from build123d import *

# Parameters (mm, degrees)
CHAMFER8_SIZE       = 0.55
BOSS_EXTRUDE3_START = 3
SKETCH8_R           = 3.9
BOSS_EXTRUDE3_DEPTH = 3


with BuildPart() as part:
    # Sketch1 → Revolve1 (revolve)
    with BuildSketch(Plane(origin=(0, 0, 0), x_dir=(1, 0, 0), z_dir=(0, 1, 0)), mode=Mode.PRIVATE) as revolve1_sk:
        Polygon((-11.4, 3.1), (11.4, 3.1), (11.4, 3.9), (4.4, 3.9), (4.4, 5), (-4.4, 5), (-4.4, 3.9), (-11.4, 3.9), align=None)
    revolve(revolve1_sk.sketch.rotate(Axis((-11.4, 0, 0), (1, 0, 0)), 180), axis=Axis((-11.4, 0, 0), (1, 0, 0)))

    # Chamfer8
    chamfer8_edges = [part.edges().sort_by_distance(p)[0] for p in [
        (4.4, 0, -3.9),
        (4.4, 0, -5),
        (-4.4, 0, -5),
        (-4.4, 0, -3.9),
    ]]
    chamfer(chamfer8_edges, length=CHAMFER8_SIZE - 0.0001)  # a hair under: the kernel refuses the full size

    # Sketch8 → Boss-Extrude3 (add)
    with BuildSketch(Plane.ZY.offset(11.4).offset(BOSS_EXTRUDE3_START)):
        Circle(SKETCH8_R)
    extrude(amount=-BOSS_EXTRUDE3_DEPTH)


solid = part.part
Design review of the part built by this model. Coordinates are the model's own, in mm. A direction names the side the tool comes from. Give positions to 0.01 mm unless a question says otherwise; leave off trailing zeros. Loops run counter-clockwise (first coordinate to the right, second up) from the corner with the lowest first, then second, coordinate; pieces in that order, holes last. Notation, with made-up numbers: M 70.5,48.25 L 106.5,48.25 A26 cw 106.5,69.25 Z; hole C -30.75,8.5 d1. An arc over 180 degrees is marked long. Answer as a JSON object with one key per item and string values.
Item 1: Machinability: for faces 4 (the face through (-14.4, 0, 0)), 5 (the face through (8.13, -2.64, -2.87)), which of the approach directions +Z, -Z, +X, -X, +Y, -Y give a long, thin tool a straight path to every point of the face, cutting with its end or side? Answer none if there is none.
Output values:
{"face 4": "+Z, -Z, -X, +Y, -Y", "face 5": "+X"}
Item 2: We need section D-D (x = -1). State the section outline as (y, z) points, and give its area (3 significant figures).
Output values:
{"outline": "C 0,0 d10; hole C 0,0 d6.2", "area": "48.3 mm2"}
Item 3: For P1, Ø1.5, axis at x = 2, z = -3.5, coming from the +Y side; P2, Ø1, axis at x = -5.5, z = 0, coming from the -Y side; P3, Ø5, axis at y = 1, z = 1, coming from the +X side; P4, Ø5, axis at x = -5.5, z = 2, coming from the -Y side, all flat-tipped, find the tip position at first contact; note any pin that passes through.
Output values:
{"P1": "stops at y = 4.18", "P2": "stops at y = -3.9", "P3": "stops at x = 11.4", "P4": "stops at y = -5"}
Item 4: Mouldability with a two-part tool opening along Y and no side actions: class faces 1 (the face through (-9.74, 2.64, -2.87)), 2 (the face through (0.16, -0.931, 2.957)), 3 (the face through (11.4, 2, 3)) as pulls with the +Y half, pulls with the -Y half, needs draft (parallel to the pull), parting line crosses it, or undercut.
Output values:
{"face 1": "parting line crosses it", "face 2": "undercut", "face 3": "needs draft"}
Item 5: We need section A-A (x = 6.75). State the section outline as (y, z) points.
Output values:
{"outline": "C 0,0 d7.8; hole C 0,0 d6.2"}
Item 6: Wall thickness on line 1 along Y through (x, z) = (-0.5, 0); line 2 along Y through (x, z) = (-5.5, 0); line 3 along X through (y, z) = (-2, 2): over which ranges is each line inside the solid? List them lowest first.
Output values:
{"line 1": "y = -5 to -3.1, 3.1 to 5", "line 2": "y = -3.9 to -3.1, 3.1 to 3.9", "line 3": "x = -14.4 to -11.4"}
